For this review, take the finished solid that the model builds, in its own axes (mm). A direction names the side the tool comes from. Coordinates: 2 decimals unless noted, no trailing zeros. Loops run counter-clockwise (first coordinate to the right, second up) from the corner with the lowest first, then second, coordinate; pieces in that order, holes last.
1. Take a section at D-D, the plane z = 35.5. State the section outline as (x, y) points.
2. Take a section at B-B, the plane x = 14. State the section outline as (y, z) points.
3. Mouldability with a two-part tool opening along X and no side actions: class faces 3 (the face through (0, -29, 26)), 4 (the face through (29.33, -12.16, 100.18)), 5 (the face through (-14.3, 21.3, 203.2)), 6 (the face through (24.227, 7.629, 100.178)) as pulls with the +X half, pulls with the -X half, needs draft (parallel to the pull), parting line crosses it, or undercut.
4. Take a section at C-C, the plane z = 74. State the section outline as (x, y) points.
5. To check wall thickness, follow probe 1 along X at (y, z) = (0, 159); probe 2 along Y at (x, z) = (1, 88.5); probe 3 along Y at (x, z) = (-22.5, 182). State the ranges of each line that lie inside material, in increasing order.
6. Clearance check with flat-ended pins moving along their axes: P1, Ø1.5, axis at y = 6, z = 136.5, coming from the +X side; P2, Ø8, axis at x = 7, y = 20, coming from the -Z side; P3, Ø5, axis at y = 30, z = 15, coming from the -X side; P4, Ø8, axis at x = 2, z = 58.5, coming from the +Y side. State where each tip first meets the part, or that it passes through.
7. Take a section at A-A, the plane y = 0. State the section outline as (x, z) points.
8. Machinability: for faces 1 (the face through (25.2, 4.9, 0)), 2 (the face through (-26, 0, 50.8)), which of the approach directions +Z, -Z, +X, -X, +Y, -Y give a long, thin tool a straight path to every point of the face, cutting with its end or side? Answer none if there is none.
```python
from build123d import *

# Parameters (mm, degrees)
SKETCH1_R           = 31.75
SKETCH1_R_2         = 25.4
BOSS_EXTRUDE1_DEPTH = 203.2
CUT_EXTRUDE1_REACH  = 210.102
SKETCH2_W           = 50.8
SKETCH2_H           = 63.5


with BuildPart() as part:
    # Sketch1 → Boss-Extrude1 (new body)
    with BuildSketch(Plane.XY):
        Circle(SKETCH1_R)
        Circle(SKETCH1_R_2, mode=Mode.SUBTRACT)
    extrude(amount=BOSS_EXTRUDE1_DEPTH)

    # Sketch2 → Cut-Extrude1 (cut, up to next)
    with BuildSketch(Plane(origin=(0, 0, 0), x_dir=(0, 0, -1), z_dir=(1, 0, 0)), mode=Mode.PRIVATE) as cut_extrude1_sk1:
        with Locations((-25.4, 0)):
            Rectangle(SKETCH2_W, SKETCH2_H)
    cut_extrude1_tool1 = extrude(cut_extrude1_sk1.sketch, amount=-CUT_EXTRUDE1_REACH, mode=Mode.PRIVATE) & part.part
    add(cut_extrude1_tool1.solids().sort_by_distance((0, 0, 25.4))[0], mode=Mode.SUBTRACT)


solid = part.part
```
Results list:
1. outline: (0, -31.75) arc R31.75 ccw to (0, 31.75) - (0, 25.4) arc R25.4 cw to (0, -25.4) - close
2. outline: (-28.5, 0) - (-21.19, 0) - (-21.19, 203.2) - (-28.5, 203.2) - close; (21.19, 0) - (28.5, 0) - (28.5, 203.2) - (21.19, 203.2) - close
3. face 3: pulls with the -X half
3. face 4: parting line crosses it
3. face 5: needs draft
3. face 6: undercut
4. outline: circle Ø63.5 at (0, 0); hole circle Ø50.8 at (0, 0)
5. probe 1: x = -31.75 to -25.4, 25.4 to 31.75
5. probe 2: y = -31.73 to -25.38, 25.38 to 31.73
5. probe 3: y = -22.4 to -11.79, 11.79 to 22.4
6. P1: stops at x = 31.31
6. P2: passes through
6. P3: stops at x = 0
6. P4: stops at y = 31.75
7. outline: (-31.75, 50.8) - (-25.4, 50.8) - (-25.4, 203.2) - (-31.75, 203.2) - close; (25.4, 0) - (31.75, 0) - (31.75, 203.2) - (25.4, 203.2) - close
8. face 1: -Z, +X, -X, +Y, -Y
8. face 2: -Z, -X, +Y, -Y
